from build123d import *

# Parameters (mm, degrees)
CROQUIS1_R              = 14.25
CROQUIS1_R_2            = 1.58
SALIENTE_EXTRUIR1_DEPTH = 6


with BuildPart() as part:
    # Croquis1 → Saliente-Extruir1 (new body)
    with BuildSketch(Plane.XY):
        with BuildLine():
            Line((110.034775737, 174.96231782), (-28.386947122, 135.91609695))
            ThreePointArc((-28.386947122, 135.91609695), (-40.514665945, 126.246932811), (-42.085274513, 110.816200885))
            Line((-42.085274513, 110.816200885), (-41.681314374, 109.494906807))
            ThreePointArc((-41.681314374, 109.494906807), (-31.943245693, 97.681684863), (-16.704181948, 96.21432992))
            Line((-16.704181948, 96.21432992), (110.034775737, 134.96231782))
            Line((110.034775737, 134.96231782), (200.034775737, 134.96231782))
            ThreePointArc((200.034775737, 134.96231782), (220.034775737, 154.96231782), (200.034775737, 174.96231782))
            Line((200.034775737, 174.96231782), (110.034775737, 174.96231782))
        make_face()
        with Locations((-12.544553236, 118.39989117)):
            Circle(CROQUIS1_R, mode=Mode.SUBTRACT)
        with Locations((200.034775737, 154.96231782)):
            Circle(CROQUIS1_R_2, mode=Mode.SUBTRACT)
        with Locations((130.034775737, 154.96231782)):
            Circle(CROQUIS1_R_2, mode=Mode.SUBTRACT)
    extrude(amount=SALIENTE_EXTRUIR1_DEPTH)


solid = part.part
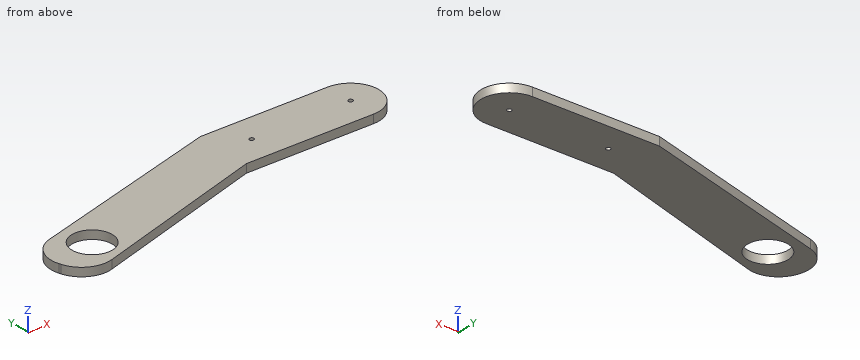
Source: CAD feature listing. Evaluate the final solid. Frame: model axes, mm. Coordinates: 2 decimals unless noted, no trailing zeros. Order: outer loops, then holes, each group sorted by start corner. A loop starts at its lowest first (then second) coordinate and runs counter-clockwise, first axis right, second up. Notation, with made-up numbers: M 21.25,-29.75 L 68.25,-29.75 A25 cw 68.25,-0.75 Z; hole C -1.75,42.5 d6. An arc over 180 degrees is marked long. Write each question's results on one line, items separated by ' | '. Start each with the question number.
Item 1: Cut plane A-A (y = 126). Return loops of the section in (x, z).
Item 2: Cut plane B-B (z = 1.5). Return loops of the section in (x, y), and give its area (3 significant figures).
Item 3: Line query: probe 1 along Y at (x, z) = (193, 5.45); probe 2 along Y at (x, z) = (-19.5, 1.25); probe 3 along Y at (x, z) = (-20.5, 3.15). Output: solid intervals per line, ascending.
Item 4: Cut plane D-D (y = 162). Return loops of the section in (x, z).
Item 5: Cut plane C-C (x = 21). Return loops of the section in (y, z).
Item 6: First-contact query: pin 1 Ø1.9 at (x, y) = (200.03, 154.96) entering from -Z; pin 2 Ø3 at (x, z) = (141, 4) entering from -Y; pin 3 Ø1 at (y, z) = (131, 1.5) entering from -X; pin 4 Ø3 at (x, z) = (26.5, 4.5) entering from -Y. Flat tips, straight axial feed; report the tip coordinate or a pass-through.
Checked values:
1) outline: M -40.65,0 L -24.6,0 L -24.6,6 L -40.65,6 Z; M -0.49,0 L 80.72,0 L 80.72,6 L -0.49,6 Z
2) outline: M -42.09,110.82 L -41.68,109.49 A20 ccw -16.7,96.21 L 110.03,134.96 L 200.03,134.96 A20 ccw 200.03,174.96 L 110.03,174.96 L -28.39,135.92 A20 ccw Z; hole C -12.54,118.4 d28.5; hole C 130.03,154.96 d3.16; hole C 200.03,154.96 d3.16 | area: 9,750 mm2
3) probe 1: y = 134.96 to 174.96 | probe 2: y = 95.57 to 105.96, 130.84 to 138.42 | probe 3: y = 95.45 to 106.58, 130.22 to 138.14
4) outline: M 64.08,0 L 218.76,0 L 218.76,6 L 64.08,6 Z
5) outline: M 107.74,0 L 149.85,0 L 149.85,6 L 107.74,6 Z
6) pin 1: passes through | pin 2: stops at y = 134.96 | pin 3: stops at x = -37.4 | pin 4: stops at y = 108.96
